Here's how the part is built. I have some questions about the finished solid (model axes, mm). A direction names the side the tool comes from. Round coordinates to 2 decimals unless told otherwise and drop trailing zeros. Loops run counter-clockwise (first coordinate to the right, second up) from the corner with the lowest first, then second, coordinate; pieces in that order, holes last. Notation, with made-up numbers: M 51,4 L 56,4 A19 ccw 56,40 Z; hole C -24,8.25 d4. An arc over 180 degrees is marked long. Answer as a JSON object with one key per item and string values.
from build123d import *

# Parameters (mm, degrees)
BOSS_EXTRUDE1_DEPTH = 3
SKETCH2_R           = 0.75
SKETCH2_R_2         = 0.5
CUT_EXTRUDE1_DEPTH  = 10


with BuildPart() as part:
    # Sketch1 → Boss-Extrude1 (new body)
    with BuildSketch(Plane(origin=(0, 0, 0), x_dir=(0, 0, -1), z_dir=(1, 0, 0))):
        Polygon((0, 0), (0, -12), (-8, -12), (-8, -62), (42, -62), (42, -12), (3, -12), (3, 0), align=None)
    extrude(amount=BOSS_EXTRUDE1_DEPTH)

    # Sketch2 → Cut-Extrude1 (cut)
    with BuildSketch(Plane.XY):
        with Locations((1.5, -2)):
            Circle(SKETCH2_R)
        with Locations((1.5, -7)):
            Circle(SKETCH2_R_2)
    extrude(amount=-CUT_EXTRUDE1_DEPTH, mode=Mode.SUBTRACT)


solid = part.part
Item 1: If we mould it in two halves opening along Y, with no side actions, what happens to faces 4 (the face through (1, -37, -42)), 5 (the face through (1, -62, -17)), 6 (the face through (1.903, -1.368, -1.479))? For each: pulls with the +Y half, pulls with the -Y half, needs draft (parallel to the pull), parting line crosses it, or undercut.
Resolved:
{"face 4": "needs draft", "face 5": "pulls with the -Y half", "face 6": "undercut"}
Item 2: I want a section at A-A, the plane y = -2. Please give me the cut outline in (x, z), then the cut area to 3 significant figures.
Resolved:
{"outline": "M 0,-3 L 0.75,-3 L 0.75,0 L 0,0 Z; M 2.25,-3 L 3,-3 L 3,0 L 2.25,0 Z", "area": "4.50 mm²"}
Item 3: I want a section at C-C, the plane z = -5. Please give me the cut outline in (x, y).
Resolved:
{"outline": "M 0,-62 L 3,-62 L 3,-12 L 0,-12 Z"}
Item 4: Please list where these lines run through material, in increasing order: probe 1 along Y at (x, z) = (1.5, -0.7); probe 2 along Z at (x, y) = (0.9, -10); probe 3 along Y at (x, z) = (1.05, -38). Write a range as from..to.
Resolved:
{"probe 1": "-62..-7.5, -6.5..-2.75, -1.25..0", "probe 2": "-3..0", "probe 3": "-62..-12"}
Item 5: I'm going to push flat-ended pins straight in: pin 1 Ø1.5 at (x, z) = (2, 5) entering from +Y; pin 2 Ø8 at (y, z) = (-14.5, 2.5) entering from -X; pin 3 Ø1.7 at (x, y) = (1.5, -2) entering from +Z. Where does each tip first touch, or does it pass through?
Resolved:
{"pin 1": "y = -12", "pin 2": "x = 0", "pin 3": "z = 0"}
Item 6: On a 3-axis mill with a long thin cutter (end or side, diameter ignored), from which of +Z, -Z, +X, -X, +Y, -Y can I reach the whole of each face in a straight line? I mean faces 1 (the face through (1, -12, -23)), 2 (the face through (1, -37, 8)), 3 (the face through (1, -12, 4)). Say none if no direction works.
Resolved:
{"face 1": "-Z, +X, -X, +Y", "face 2": "+Z, +X, -X, +Y, -Y", "face 3": "+Z, +X, -X, +Y"}
Item 7: I want a section at B-B, the plane x = 1.5. Please give me the cut outline in (y, z).
Resolved:
{"outline": "M -62,-42 L -12,-42 L -12,-3 L -7.5,-3 L -7.5,0 L -12,0 L -12,8 L -62,8 Z; M -6.5,-3 L -2.75,-3 L -2.75,0 L -6.5,0 Z; M -1.25,-3 L 0,-3 L 0,0 L -1.25,0 Z"}
